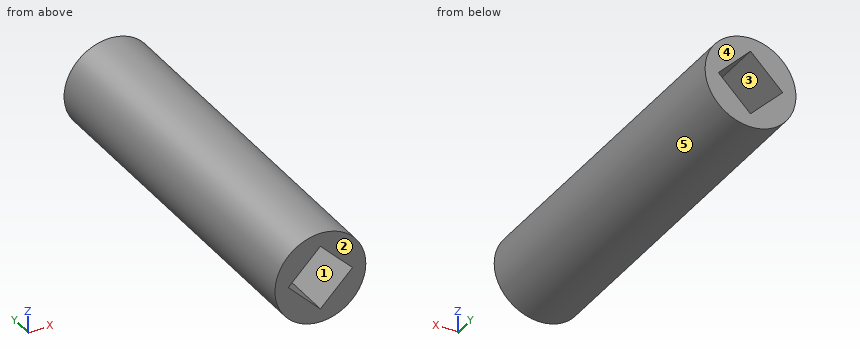
```python
from build123d import *

# Parameters (mm, degrees)
F0_R     = 12.7
F1_DEPTH = 101.6
F3_DEPTH = 27.94
F5_DEPTH = 27.94
F7_R     = 9.525
F8_DEPTH = 45.72


with BuildPart() as f1:
    # F0 (on Front) → F1 (new body)
    with BuildSketch(Plane.XZ):
        Circle(F0_R)
    extrude(amount=F1_DEPTH)

    # F2 (on face) → F3 (cut)
    with BuildSketch(Plane.XZ.offset(101.6)):
        Polygon((0, -8.980256), (8.980256, 0), (0, 8.980256), (-8.980256, 0), align=None)
    extrude(amount=-F3_DEPTH, mode=Mode.SUBTRACT)

    # F4 (on face) → F5 (cut)
    with BuildSketch(Plane(origin=(0, 0, 0), x_dir=(-1, 0, 0), z_dir=(0, 1, 0))):
        Polygon((0, -8.980256), (8.980256, 0), (0, 8.980256), (-8.980256, 0), align=None)
    extrude(amount=-F5_DEPTH, mode=Mode.SUBTRACT)

    # F7 (on offset) → F8 (cut)
    with BuildSketch(Plane.XZ.offset(27.94)):
        Circle(F7_R)
    extrude(amount=F8_DEPTH, mode=Mode.SUBTRACT)


solid = f1.part
```
Geometry: final body of the model. Coordinates: model frame, mm. Face numbers are marked on the shaded views. A direction names the side the tool comes from. Round coordinates to 2 decimals unless told otherwise and drop trailing zeros. Order: outer loops, then holes, each group sorted by start corner. A loop starts at its lowest first (then second) coordinate and runs counter-clockwise, first axis right, second up. Notation, with made-up numbers: (14.5, 89) - (53.5, 89) arc R6 ccw to (53.5, 94) - close; hole circle Ø1 at (-21, 71). An arc over 180 degrees is marked (long way). Use CSV: the item, a comma, the result in double quotes. Start each with the question number.
Q1. Section query A-A (x = 5). Return loops of the section in (y, z).
Q2. Mould query, pull axis X, two halves, no side actions, for the marked faces 3, 4 and 5. Classes: +X half, -X half, draft (parallel to the pull), parting line (faces both ways), or undercut.
Q3. Section query C-C (y = -90.5). Return loops of the section in (x, z).
Q4. Section query B-B (z = -6.5). Return loops of the section in (x, y).
Q5. Section query D-D (y = -44). Return loops of the section in (x, z) (3 decimals), and give its area (3 significant figures).
Q6. Access query for the marked faces 1 and 2. Directions: +Z, -Z, +X, -X, +Y, -Y. A direction counts if a zero-diameter tool reaches every point of the face in a straight line with its end or side. Return the directions, or none.
Q7. Material intervals for line 1 along Z through (x, y) = (0, -56) (3 decimals); line 2 along Y through (x, z) = (-7.25, -2); line 3 along X through (y, z) = (-30.5, 6.75), sorted ascending. Write a range as from..to.
Q8. First-contact query: pin 1 (3 mm diameter, centred on x = 4, y = -82, fed in from +Z); pin 2 (12 mm diameter, centred on y = -55, z = 7, fed in from -X); pin 3 (2 mm diameter, centred on y = -73, z = -10, fed in from -X). Flat tips, straight axial feed; report the tip coordinate or a pass-through.
Result set:
1,outline,"(-101.6, -11.67) - (0, -11.67) - (0, -3.98) - (-27.94, -3.98) - (-27.94, -8.11) - (-73.66, -8.11) - (-73.66, -3.98) - (-101.6, -3.98) - close; (-101.6, 3.98) - (-73.66, 3.98) - (-73.66, 8.11) - (-27.94, 8.11) - (-27.94, 3.98) - (0, 3.98) - (0, 11.67) - (-101.6, 11.67) - close"
2,face 3,"undercut"
2,face 4,"draft"
2,face 5,"parting line"
3,outline,"circle Ø25.4 at (0, 0); hole (-8.98, 0) - (0, -8.98) - (8.98, 0) - (0, 8.98) - close"
4,outline,"(-10.91, -101.6) - (-2.48, -101.6) - (-2.48, -73.66) - (-6.96, -73.66) - (-6.96, -27.94) - (-2.48, -27.94) - (-2.48, 0) - (-10.91, 0) - close; (2.48, -101.6) - (10.91, -101.6) - (10.91, 0) - (2.48, 0) - (2.48, -27.94) - (6.96, -27.94) - (6.96, -73.66) - (2.48, -73.66) - close"
5,outline,"circle Ø25.4 at (0, 0); hole circle Ø19.05 at (0, 0)"
5,area,"222 mm2"
6,face 1,"+Y, -Y"
6,face 2,"+Z, -Z, +X, -X, -Y"
7,line 1,"z = -12.7..-9.525, 9.525..12.7"
7,line 2,"y = -101.6..-73.66, -27.94..0"
7,line 3,"x = -10.76..-6.72, 6.72..10.76"
8,pin 1,"stops at z = 12.45"
8,pin 2,"stops at x = -12.66"
8,pin 3,"stops at x = -8.96"
